```python
from build123d import *

# Parameters (mm, degrees)
F0_R     = 10.3251
F1_DEPTH = 7.9375
F2_R     = 9.92251
F3_DEPTH = 88.9
F5_DEPTH = 57.15
F6_R     = 12.7
F7_R     = 12.7


with BuildPart() as f1:
    # F0 (on Top) → F1 (new body)
    with BuildSketch(Plane.XY):
        with BuildLine():
            Line((0, 44.45), (0, -44.45))
            Line((0, -44.45), (57.15, -44.45))
            Line((57.15, -44.45), (57.15, -28.575))
            ThreePointArc((57.15, -28.575), (59.009872, -24.084872), (63.5, -22.225))
            Line((63.5, -22.225), (111.125, -22.225))
            ThreePointArc((111.125, -22.225), (133.35, 0), (111.125, 22.225))
            Line((111.125, 22.225), (63.5, 22.225))
            ThreePointArc((63.5, 22.225), (59.009872, 24.084872), (57.15, 28.575))
            Line((57.15, 28.575), (57.15, 44.45))
            Line((57.15, 44.45), (0, 44.45))
        make_face()
        with Locations((73.025, 0)):
            Circle(F0_R, mode=Mode.SUBTRACT)
        with Locations((111.125, 0)):
            Circle(F0_R, mode=Mode.SUBTRACT)
    extrude(amount=F1_DEPTH)

    # F2 (on face) → F3 (join)
    with BuildSketch(Plane.XZ.offset(44.45)):
        with BuildLine():
            Line((0, 52.3875), (0, 7.9375))
            Line((0, 7.9375), (57.15, 7.9375))
            Line((57.15, 7.9375), (57.15, 52.3875))
            ThreePointArc((57.15, 52.3875), (28.575, 80.9625), (0, 52.3875))
        make_face()
        with Locations((28.575, 52.3875)):
            Circle(F2_R, mode=Mode.SUBTRACT)
    extrude(amount=-F3_DEPTH)

    # F4 (on face) → F5 (cut)
    with BuildSketch(Plane(origin=(0, 0, 0), x_dir=(0, -1, 0), z_dir=(-1, 0, 0))):
        with BuildLine():
            ThreePointArc((-36.5125, 12.7), (-35.117596, 9.332404), (-31.75, 7.9375))
            Line((-31.75, 7.9375), (31.75, 7.9375))
            ThreePointArc((31.75, 7.9375), (35.117596, 9.332404), (36.5125, 12.7))
            Line((36.5125, 12.7), (36.5125, 84.1375))
            Line((36.5125, 84.1375), (-36.5125, 84.1375))
            Line((-36.5125, 84.1375), (-36.5125, 12.7))
        make_face()
    extrude(amount=-F5_DEPTH, mode=Mode.SUBTRACT)

    # F6
    f6_edges = [f1.edges().sort_by_distance(p)[0] for p in [
        (28.575, 44.45, 0),
    ]]
    fillet(f6_edges, radius=F6_R)

    # F7
    f7_edges = [f1.edges().sort_by_distance(p)[0] for p in [
        (28.575, -44.45, 0),
    ]]
    fillet(f7_edges, radius=F7_R)


solid = f1.part
```
Can you work these out from the model? Positions are in its coordinate system, mm. A direction names the side the tool comes from. Coordinates: 2 decimals unless noted, no trailing zeros. Loops run counter-clockwise (first coordinate to the right, second up) from the corner with the lowest first, then second, coordinate; pieces in that order, holes last.
1) Which directions (+Z, -Z, +X, -X, +Y, -Y) give clear straight access to the entire face, cutting with the end or side of a thin tool? Please do faces 1 (the flat face through (88, 22.225, 4)), 2 (the cylindrical face through (62.71, 0.45, 3.91)), 3 (the cylindrical face through (28, 41, 4)), 4 (the flat face through (51, 0, 7.938)), 5 (the flat face through (87, -22.225, 4)).
2) Imagine slicing it at A-A on z = 23.5. List the corners of the cut face in (x, y) for me, plus the area to 3 significant figures.
3) Imagine slicing it at B-B on y = 6. List the corners of the cut face in (x, z) for me, plus the area to 3 significant figures.
4) For pin 1 (3 mm diameter, centred on x = 44, y = 33, fed in from +Z); pin 2 (17.5 mm diameter, centred on y = -40, z = 23.5, fed in from +X); pin 3 (8.5 mm diameter, centred on x = 76.5, z = 3.5, fed in from +Y) (3 decimals), each with a flat end and sliding along its axis, tell me the tip position at first contact or that it passes through.
5) Imagine slicing it at C-C on x = 105.5. List the corners of the cut face in (y, z) for me (1 decimal).
6) Thinking about a two-plate mould opening in X: for faces 6 (the cylindrical face through (59.06, 24.036, 3.913)), 7 (the cylindrical face through (120.973, 3.101, 3.913)), 8 (the flat face through (28, 36.512, 40)), which applies, pulls with the +X half, pulls with the -X half, needs draft (parallel to the pull), parting line crosses it, or undercut?
7) Imagine slicing it at D-D on z = 47.5. List the corners of the cut face in (x, y) for me.
8) I need wall thicknesses on probe 1 along Y at (x, z) = (8.5, 26); probe 2 along Z at (x, y) = (111, 20.5); probe 3 along X at (y, z) = (41, 22). Which ranges of each line are inside material? Lowest first, please.
Completed:
1. face 1: +Z, -Z, +X, +Y
1. face 2: +Z, -Z
1. face 3: -Z, +X, -X, +Y
1. face 4: +Z, +X, -X
1. face 5: +Z, -Z, +X, -Y
2. outline: (0, -44.45) - (57.15, -44.45) - (57.15, -36.51) - (0, -36.51) - close; (0, 36.51) - (57.15, 36.51) - (57.15, 44.45) - (0, 44.45) - close
2. area: 907 mm2
3. outline: (0, 0) - (64.62, 0) - (64.62, 7.94) - (0, 7.94) - close; (81.43, 0) - (102.72, 0) - (102.72, 7.94) - (81.43, 7.94) - close; (119.53, 0) - (132.52, 0) - (132.52, 7.94) - (119.53, 7.94) - close
3. area: 785 mm2
4. pin 1: stops at z = 8.81
4. pin 2: stops at x = 57.15
4. pin 3: stops at y = 22.225
5. outline: (-22.2, 0) - (-8.7, 0) - (-8.7, 7.9) - (-22.2, 7.9) - close; (8.7, 0) - (22.2, 0) - (22.2, 7.9) - (8.7, 7.9) - close
6. face 6: pulls with the +X half
6. face 7: undercut
6. face 8: needs draft
7. outline: (0, -44.45) - (19.94, -44.45) - (19.94, -36.51) - (0, -36.51) - close; (0, 36.51) - (19.94, 36.51) - (19.94, 44.45) - (0, 44.45) - close; (37.21, -44.45) - (57.15, -44.45) - (57.15, -36.51) - (37.21, -36.51) - close; (37.21, 36.51) - (57.15, 36.51) - (57.15, 44.45) - (37.21, 44.45) - close
8. probe 1: y = -44.45 to -36.51, 36.51 to 44.45
8. probe 2: z = 0 to 7.94
8. probe 3: x = 0 to 57.15
